from build123d import *

# Parameters (mm, degrees)
BOSS_EXTRUDE1_DEPTH = 3
SKETCH4_W           = 15.6
SKETCH4_H           = 1
CUT_EXTRUDE1_DEPTH  = 5
BOSS_EXTRUDE3_DEPTH = 3


with BuildPart() as part:
    # Sketch1 → Boss-Extrude1 (new body)
    with BuildSketch(Plane.XY):
        Polygon((29.821727019, -20.842278002), (-26.378272981, -20.842278002), (-29.378272981, -20.842278002), (-29.378272981, -10.842278002), (-26.378272981, -10.842278002), (-23.978272981, -10.842278002), (-23.978272981, -16.442278002), (-7.378272981, -16.442278002), (-7.378272981, -10.842278002), (-3.778272981, -10.842278002), (-3.778272981, -14.842278002), (9.821727019, -14.842278002), (9.821727019, -10.842278002), (14.221727019, -10.842278002), (14.221727019, -14.842278002), (27.821727019, -14.842278002), (27.821727019, -10.842278002), (29.821727019, -10.842278002), (32.821727019, -10.842278002), (32.821727019, -20.842278002), align=None)
    extrude(amount=BOSS_EXTRUDE1_DEPTH)

    # Sketch4 → Cut-Extrude1 (cut)
    with BuildSketch(Plane(origin=(0, -10.842278002, 0), x_dir=(1, 0, 0), z_dir=(0, 1, 0))):
        with Locations((3.021727019, -1.5)):
            Rectangle(SKETCH4_W, SKETCH4_H)
        with Locations((21.021727019, -1.5)):
            Rectangle(SKETCH4_W, SKETCH4_H)
    extrude(amount=-CUT_EXTRUDE1_DEPTH, mode=Mode.SUBTRACT)

    # Sketch5 → Boss-Extrude3 (add)
    with BuildSketch(Plane(origin=(0, 0, 0), x_dir=(-1, 0, 0), z_dir=(0, 0, -1))):
        Polygon((-32.821727019, -10.842278002), (-32.821727019, -20.842278002), (29.378272981, -20.842278002), (29.378272981, -10.842278002), (26.378272981, -10.842278002), (26.378272981, -17.842278002), (-29.821727019, -17.842278002), (-29.821727019, -10.842278002), align=None)
    extrude(amount=BOSS_EXTRUDE3_DEPTH)


solid = part.part
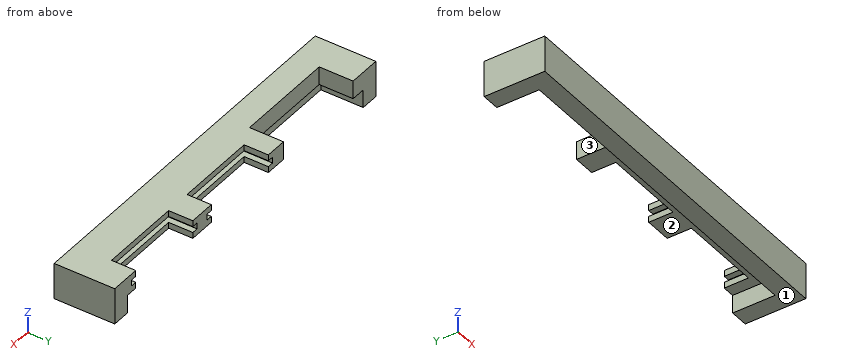
Geometry check sheet. Reference: the model listing, model coordinates, mm. Face numbers are marked on the shaded views. A direction names the side the tool comes from. Give positions to 0.01 mm unless a question says otherwise; leave off trailing zeros. Order: outer loops, then holes, each group sorted by start corner. A loop starts at its lowest first (then second) coordinate and runs counter-clockwise, first axis right, second up. Notation, with made-up numbers: (3, 23) - (59, 23) arc R7 ccw to (59, 34) - close; hole circle Ø4 at (18.25, -10.75). An arc over 180 degrees is marked (long way). Use one line per item in the form item = value.
1) Depth check by flat-ended pin: pin 1 Ø0.9 at (x, z) = (-19.5, 2) entering from +Y; pin 2 Ø5.5 at (x, y) = (20.5, -13) entering from -Z. Enter the tip coordinate at first touch or a pass-through.
Working result:
pin_1 = -16.44
pin_2 = 0
2) Access from +Z, -Z, +X, -X, +Y, -Y to the whole of each face (thin tool, end or side, straight path). Record for the marked faces 1, 2 and 3.
Working result:
face_1 = -Z, +X, -X, +Y, -Y
face_2 = -Z, +Y
face_3 = +Z, -Z, +Y
3) Sectioned sample at A-A (z = -1.6). Record the boundary of the cut face in (x, y).
Working result:
outline = (-29.38, -20.84) - (32.82, -20.84) - (32.82, -10.84) - (29.82, -10.84) - (29.82, -17.84) - (-26.38, -17.84) - (-26.38, -10.84) - (-29.38, -10.84) - close
4) Sectioned sample at D-D (y = -13.5). Count the separate pieces of the cut face and the enclosed holes in it, and give its area (3 significant figures).
Working result:
separate_pieces = 4
enclosed_holes = 0
area = 69.2 mm^2
5) Sectioned sample at C-C (x = 3). Record the boundary of the cut face in (y, z), and give its area (3 significant figures).
Working result:
outline = (-20.84, -3) - (-17.84, -3) - (-17.84, 0) - (-14.84, 0) - (-14.84, 1) - (-15.84, 1) - (-15.84, 2) - (-14.84, 2) - (-14.84, 3) - (-20.84, 3) - close
area = 26.0 mm^2
6) Material ranges on probe 1 along X at (y, z) = (-11.25, 1.9); probe 2 along X at (y, z) = (-14.5, 0.05); probe 3 along X at (y, z) = (-12, -0.4), recorded low to high. Write a range as from..to.
Working result:
probe_1 = -29.38..-23.98, -7.38..-4.78, 10.82..13.22, 28.82..32.82
probe_2 = -29.38..-23.98, -7.38..-3.78, 9.82..14.22, 27.82..32.82
probe_3 = -29.38..-26.38, 29.82..32.82
7) Sectioned sample at B-B (y = -17). Record the boundary of the cut face in (x, z), and give its area (3 significant figures).
Working result:
outline = (-29.38, -3) - (-26.38, -3) - (-26.38, 0) - (29.82, 0) - (29.82, -3) - (32.82, -3) - (32.82, 3) - (-29.38, 3) - close
area = 205 mm^2
